For this review, take the finished solid that the model builds, in its own axes (mm). A direction names the side the tool comes from. Coordinates: 2 decimals unless noted, no trailing zeros. Loops run counter-clockwise (first coordinate to the right, second up) from the corner with the lowest first, then second, coordinate; pieces in that order, holes last. Notation, with made-up numbers: (0, 54.25) - (12, 54.25) arc R16 cw to (12, 65.25) - close; hole circle Ø11 at (82.5, 42). An arc over 180 degrees is marked (long way). Use one line per item in the form item = value. Start each with the question number.
1. Add section A-A on y = 0. Give the boundary of the cut face in (x, z).
2. To check wall thickness, follow probe 1 along Y at (x, z) = (0, 8.25); probe 2 along Y at (x, z) = (-10.5, 3); probe 3 along Y at (x, z) = (-17, 19.75). State the ranges of each line that lie inside material, in increasing order.
3. Machinability: for faces 1 (the face through (19, -19, 2)), 2 (the face through (1.327, 19.723, 11.154)), which of the approach directions +Z, -Z, +X, -X, +Y, -Y give a long, thin tool a straight path to every point of the face, cutting with its end or side? Answer none if there is none.
4. For pin 1 Ø10 at (x, z) = (-3.5, 2.5) entering from -Y; pin 2 Ø2 at (y, z) = (-16, 3.5) entering from -X; pin 3 Ø1.5 at (x, z) = (-10, 16) entering from +Y, all flat-tipped, find the tip position at first contact; note any pin that passes through.
5. Draft analysis for pull direction Y (two halves, no side actions). For faces 3 (the face through (12, -6, 0)), 4 (the face through (-12.919, -14.783, 11.154)), 5 (the face through (26.327, -10.916, 0.986)), state which applies: +Y half, -Y half, draft (parallel to the pull), parting line (faces both ways), or undercut.
6. Add section D-D on x = -21. Give the boundary of the cut face in (y, z).
7. Add section B-B on z = 11.75. Count the separate pieces of the cut face and the enclosed holes in it, and give its area (3 significant figures).
```python
from build123d import *

# Parameters (mm, degrees)
F0_R     = 26.5
F0_R_2   = 12.9
F1_DEPTH = 22
F0_R_3   = 28.5
F2_DEPTH = 2
F4_DEPTH = 22
F5_COUNT = 8


with BuildPart() as f1:
    # F0 (on Top) → F1 (new body)
    with BuildSketch(Plane.XY):
        Circle(F0_R)
        Circle(F0_R_2, mode=Mode.SUBTRACT)
    extrude(amount=F1_DEPTH)

    # F0 (on Top) → F2 (join)
    with BuildSketch(Plane.XY):
        Circle(F0_R_3)
        Circle(F0_R, mode=Mode.SUBTRACT)
    extrude(amount=F2_DEPTH)


with BuildPart() as f4:
    # F3 (on face) → F4 (new body, through all)
    with BuildSketch(Plane.XY.offset(22)):
        with BuildLine():
            ThreePointArc((1.644295, -24.44476), (9.375744, -22.635049), (16.122363, -18.447748))
            Line((16.122363, -18.447748), (9.805029, -11.219243))
            ThreePointArc((9.805029, -11.219243), (5.701983, -13.765805), (1, -14.866405))
            Line((1, -14.866405), (1.644295, -24.44476))
        make_face()
    extrude(amount=-F4_DEPTH)


with BuildPart() as f5_1:
    # F5: instance of F4
    add(f4.part.rotate(Axis((0, 0, 0), (0, 0, -1)), 1 * 360 / F5_COUNT))


with BuildPart() as f5_2:
    # F5: instance of F4
    add(f4.part.rotate(Axis((0, 0, 0), (0, 0, -1)), 2 * 360 / F5_COUNT))


with BuildPart() as f5_3:
    # F5: instance of F4
    add(f4.part.rotate(Axis((0, 0, 0), (0, 0, -1)), 3 * 360 / F5_COUNT))


with BuildPart() as f5_4:
    # F5: instance of F4
    add(f4.part.rotate(Axis((0, 0, 0), (0, 0, -1)), 4 * 360 / F5_COUNT))


with BuildPart() as f5_5:
    # F5: instance of F4
    add(f4.part.rotate(Axis((0, 0, 0), (0, 0, -1)), 5 * 360 / F5_COUNT))


with BuildPart() as f5_6:
    # F5: instance of F4
    add(f4.part.rotate(Axis((0, 0, 0), (0, 0, -1)), 6 * 360 / F5_COUNT))


with BuildPart() as f5_7:
    # F5: instance of F4
    add(f4.part.rotate(Axis((0, 0, 0), (0, 0, -1)), 7 * 360 / F5_COUNT))


with BuildPart() as f1_1:
    add(f1.part)

    # F6: cut F4, F5_7, F5_6, F5_5, F5_4, F5_3, F5_2, F5_1
    add(f4.part, mode=Mode.SUBTRACT)
    add(f5_7.part, mode=Mode.SUBTRACT)
    add(f5_6.part, mode=Mode.SUBTRACT)
    add(f5_5.part, mode=Mode.SUBTRACT)
    add(f5_4.part, mode=Mode.SUBTRACT)
    add(f5_3.part, mode=Mode.SUBTRACT)
    add(f5_2.part, mode=Mode.SUBTRACT)
    add(f5_1.part, mode=Mode.SUBTRACT)


solid = f1_1.part
```
Conclusion:
q1.outline = (-28.5, 0) - (-12.9, 0) - (-12.9, 22) - (-26.5, 22) - (-26.5, 2) - (-28.5, 2) - close; (12.9, 0) - (28.5, 0) - (28.5, 2) - (26.5, 2) - (26.5, 22) - (12.9, 22) - close
q2.probe_1 = -26.5 to -12.9, 12.9 to 26.5
q2.probe_2 = -24.33 to -22.14, -12.01 to -7.49, 7.49 to 12.01, 22.14 to 24.33
q2.probe_3 = -20.33 to -14.86, -1.14 to 1.14, 14.86 to 20.33
q3.face_1 = +Z
q3.face_2 = +Z, -Z
q4.pin_1 = -28.5
q4.pin_2 = -21.85
q4.pin_3 = 24.83
q5.face_3 = draft
q5.face_4 = undercut
q5.face_5 = parting line
q6.outline = (-19.27, 0) - (-12.62, 0) - (-12.62, 22) - (-16.16, 22) - (-16.16, 2) - (-19.27, 2) - close; (-1.41, 0) - (1.41, 0) - (1.41, 22) - (-1.41, 22) - close; (12.62, 0) - (19.27, 0) - (19.27, 2) - (16.16, 2) - (16.16, 22) - (12.62, 22) - close
q7.separate_pieces = 1
q7.enclosed_holes = 9
q7.area = 698 mm^2
